Could you check a few things on this drawing? It's one solid part, dimensions in mm from its lowest x, y, z. Give positions to 0.01 mm unless a question says otherwise; leave off trailing zeros. Loops run counter-clockwise (first coordinate to the right, second up) from the corner with the lowest first, then second, coordinate; pieces in that order, holes last.
1. Imagine slicing it at D-D (z = 156). List the corners of the cut face in (x, y) for me.
2. Imagine slicing it at B-B (x = 119). List the corners of the cut face in (y, z) for me (1 decimal), plus the area to 3 significant figures.
3. For P1, Ø2, axis at x = 60.5, y = 1, coming from the +Z side; P2, Ø1.5, axis at x = 41, y = 0.5, coming from the +Z side (1 decimal); P3, Ø2, axis at x = 83, z = 155.5, coming from the -Y side; P4, Ø1.5, axis at x = 88.5, y = 3, coming from the +Z side, each with a flat end and sliding along its axis, tell me the tip position at first contact or that it passes through.
4. I need wall thicknesses on line 1 along Z through (x, y) = (115, 4.55) (1 decimal); line 2 along X through (y, z) = (0.6, 88.5) (1 decimal); line 3 along Z through (x, y) = (104, 1.4) (1 decimal). Which ranges of each line are inside material? Lowest first, please.
5. Imagine slicing it at C-C (y = 3.45). List the corners of the cut face in (x, z) for me (1 decimal).
6. Imagine slicing it at A-A (z = 89). List the corners of the cut face in (x, y) for me (1 decimal), plus the area to 3 significant figures.
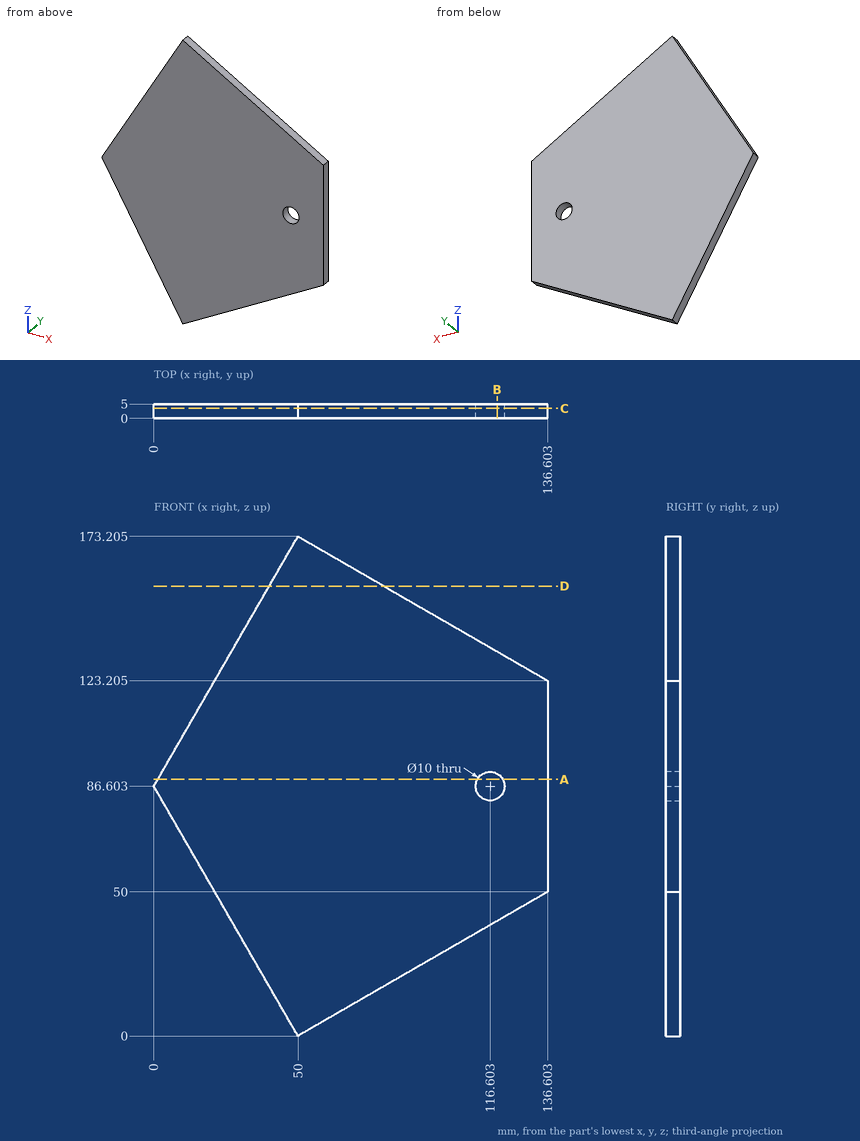
Derived:
1. outline: (40.07, 0) - (79.8, 0) - (79.8, 5) - (40.07, 5) - close
2. outline: (0, 39.8) - (5, 39.8) - (5, 82.2) - (0, 82.2) - close; (0, 91) - (5, 91) - (5, 133.4) - (0, 133.4) - close
2. area: 424 mm2
3. P1: stops at z = 167.72
3. P2: stops at z = 158.9
3. P3: passes through
3. P4: stops at z = 151.41
4. line 1: z = 37.5 to 81.9, 91.3 to 135.7
4. line 2: x = 1.1 to 112, 121.2 to 136.6
4. line 3: z = 31.2 to 142
5. outline: (0, 86.6) - (50, 0) - (136.6, 50) - (136.6, 123.2) - (50, 173.2) - close; hole circle Ø10 at (116.6, 86.6)
6. outline: (1.4, 0) - (112.2, 0) - (112.2, 5) - (1.4, 5) - close; (121, 0) - (136.6, 0) - (136.6, 5) - (121, 5) - close
6. area: 632 mm2
